The listing builds one solid part. Answer for the finished solid, in the listing's coordinates (mm). Face numbers are marked on the shaded views. A direction names the side the tool comes from. Coordinates: 2 decimals unless noted, no trailing zeros. Write each loop counter-clockwise with the first axis right and the second up, starting at its lowest first coordinate (ties: lowest second). Pieces come first, ordered by that corner, then holes. Notation, with made-up numbers: M -35.5,60 L -28.5,60 A35 cw -28.5,96 Z; hole C 89,26 d4. An arc over 180 degrees is marked long. Answer as CSV lines item,"result".
```python
from build123d import *

# Parameters (mm, degrees)
BOSS_EXTRUDE1_DEPTH = 20
SKETCH3_W           = 4.5
SKETCH3_H           = 90
CUT_EXTRUDE2_DEPTH  = 10
SKETCH4_R           = 1.5
SKETCH4_R_2         = 2
CUT_EXTRUDE3_DEPTH  = 10
CHAMFER1_SIZE       = 1
FILLET1_R           = 22
FILLET2_R           = 20


with BuildPart() as part:
    # Sketch1 → Boss-Extrude1 (new, symmetric)
    with BuildSketch(Plane(origin=(0, 0, 0), x_dir=(0, 0, -1), z_dir=(1, 0, 0))):
        Polygon((0, 0), (150, 0), (150, 3), (150, 75), (120, 75), (0, 75), align=None)
        Polygon((144, 5), (5, 5), (5, 70), (120, 70), (144, 70), align=None, mode=Mode.SUBTRACT)
    extrude(amount=BOSS_EXTRUDE1_DEPTH, both=True)

    # Sketch3 → Cut-Extrude2 (cut)
    with BuildSketch(Plane.XZ):
        with Locations((0, -75)):
            Rectangle(SKETCH3_W, SKETCH3_H)
    extrude(amount=-CUT_EXTRUDE2_DEPTH, mode=Mode.SUBTRACT)

    # Sketch4 → Cut-Extrude3 (cut)
    with BuildSketch(Plane(origin=(0, 75, 0), x_dir=(1, 0, 0), z_dir=(0, 1, 0))):
        with Locations(Location((-4.242640687, 76.742640687, 0), (0, 0, 270))):
            Circle(SKETCH4_R)
        with Locations(Location((4.242640687, 76.742640687, 0), (0, 0, 270))):
            Circle(SKETCH4_R)
        with Locations(Location((4.242640687, 68.257359313, 0), (0, 0, 270))):
            Circle(SKETCH4_R)
        with Locations(Location((-4.242640687, 68.257359313, 0), (0, 0, 270))):
            Circle(SKETCH4_R)
        with Locations(Location((0, 72.5, 0), (0, 0, 270))):
            Circle(SKETCH4_R_2)
    extrude(amount=-CUT_EXTRUDE3_DEPTH, mode=Mode.SUBTRACT)

    # Chamfer1
    chamfer1_edges = [part.edges().sort_by_distance(p)[0] for p in [
        (-4.242640687, 75, -78.242640687),
        (4.242640687, 75, -78.242640687),
        (4.242640687, 75, -69.757359313),
        (-4.242640687, 75, -69.757359313),
    ]]
    chamfer(chamfer1_edges, length=CHAMFER1_SIZE)

    # Fillet1
    fillet1_edges = [part.edges().sort_by_distance(p)[0] for p in [
        (0, 70, -5),
        (0, 5, -5),
        (0, 5, -144),
        (0, 70, -144),
    ]]
    fillet(fillet1_edges, radius=FILLET1_R)

    # Fillet2
    fillet2_edges = [part.edges().sort_by_distance(p)[0] for p in [
        (0, 75, 0),
        (0, 75, -150),
        (0, 0, -150),
        (0, 0, 0),
    ]]
    fillet(fillet2_edges, radius=FILLET2_R)


solid = part.part
```
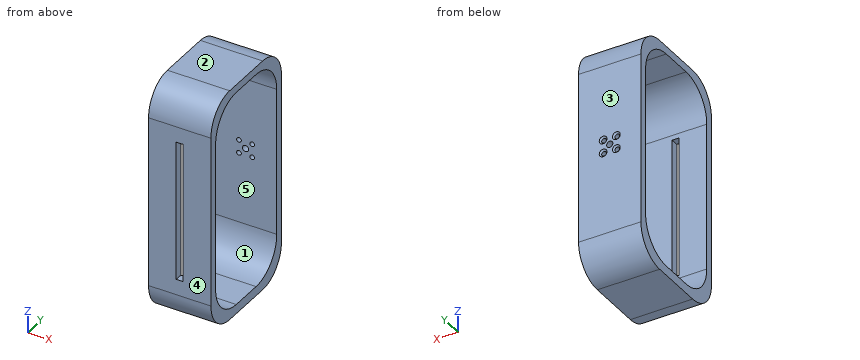
Q1. For the marked faces 4 and 5, determine the directions among +Z, -Z, +X, -X, +Y, -Y from which every point of the face is accessible in a straight line to the end or side of a thin tool.
Output:
face 4,"+Z, -Z, +X, -X, -Y"
face 5,"+X, -X"
Q2. Straight lines are drawn through the part: line 1 (Y direction, x = -7, z = -42.5); line 2 (Z direction, x = -3.5, y = 34); line 3 (X direction, y = 4, z = -30.5). For each, find the intervals that lie inside material, in ascending order.
Output:
line 1,"0 to 5, 70 to 75"
line 2,"-150 to -144, -5 to 0"
line 3,"-20 to -2.25, 2.25 to 20"
Q3. Find section B-B (z = -72.5). Give the vertices of the cut face in (x, y), and give its area (4 significant figures).
Output:
outline,"M -20,0 L -2.25,0 L -2.25,5 L -20,5 Z; M -20,70 L -2,70 L -2,75 L -20,75 Z; M 2,70 L 20,70 L 20,75 L 2,75 Z; M 2.25,0 L 20,0 L 20,5 L 2.25,5 Z"
area,"357.5 mm2"
Q4. Flat-ended cylindrical pins translate along their axes: pin 1 Ø2 at (x, y) = (-0.5, 2) entering from -Z; pin 2 Ø3 at (x, z) = (0.5, -82) entering from -Y; pin 3 Ø2 at (x, y) = (0, 3.5) entering from +Z. Find the tip coordinate at first contact, or state that the pin passes through.
Output:
pin 1,"z = -140.54"
pin 2,"y = 70"
pin 3,"z = -7.36"
Q5. The mould has two halves that part along Z. Classify the marked faces 1, 2 and 3: pulls with the +Z half, pulls with the -Z half, needs draft (parallel to the pull), parting line crosses it, or undercut.
Output:
face 1,"undercut"
face 2,"pulls with the +Z half"
face 3,"needs draft"
Q6. Find section A-A (y = 38). Give the vertices of the cut face in (x, z).
Output:
outline,"M -20,-150 L 20,-150 L 20,-144 L -20,-144 Z; M -20,-5 L 20,-5 L 20,0 L -20,0 Z"
Q7. Find section D-D (z = -55.5). Give the vertices of the cut face in (x, y), and give its area (4 significant figures).
Output:
outline,"M -20,0 L -2.25,0 L -2.25,5 L -20,5 Z; M -20,70 L 20,70 L 20,75 L -20,75 Z; M 2.25,0 L 20,0 L 20,5 L 2.25,5 Z"
area,"377.5 mm2"
Q8. Find section C-C (x = 0). Give the vertices of the cut face in (y, z), and give its area (3 significant figures).
Output:
outline,"M 0,-130 A20 ccw 20,-150 L 55,-150 A20 ccw 75,-130 L 75,-74.5 L 70,-74.5 L 70,-122 A22 cw 48,-144 L 27,-144 A22 cw 5,-122 L 5,-120 L 0,-120 Z; M 0,-30 L 5,-30 L 5,-27 A22 cw 27,-5 L 48,-5 A22 cw 70,-27 L 70,-70.5 L 75,-70.5 L 75,-20 A20 ccw 55,0 L 20,0 A20 ccw 0,-20 Z"
area,"1,820 mm2"
